Build history of the part. All positions in model axes, mm. Give positions to 0.01 mm unless a question says otherwise; leave off trailing zeros. Loops run counter-clockwise (first coordinate to the right, second up) from the corner with the lowest first, then second, coordinate; pieces in that order, holes last. Notation, with made-up numbers: (26, 68) - (67, 68) arc R24 ccw to (67, 99) - close; hole circle Ø9 at (17.25, 85.25). An arc over 180 degrees is marked (long way). Return JSON: item names as keys, results as strings. Group by question number.
1) Slice it at C-C (y = -4). List the corners of the cut face in (x, z), and give its area (3 significant figures).
2) Slice it at D-D (x = 1.3). Count the separate pieces of the cut face and the enclosed holes in it, and give its area (3 significant figures).
3) Drop flat-ended pins along their axis: pin 1 (20.5 mm diameter, centred on y = -34, z = 0, fed in from -X); pin 2 (1.5 mm diameter, centred on x = 1, y = 31, fed in from -Z); pin 3 (1 mm diameter, centred on x = 0.5, y = 7.5, fed in from -Z). Give the stop position or say it passes through.
4) Drill centre lines: probe 1 along Z at (x, y) = (0.8, -14); probe 2 along Z at (x, y) = (1.15, 44.5); probe 3 along Y at (x, z) = (2.3, 0). Where is each one in solid material? Low to high. Write a range as from..to.
5) Slice it at A-A (y = 42). List the corners of the cut face in (x, z).
6) Slice it at B-B (y = -38). List the corners of the cut face in (x, z), and give its area (3 significant figures).
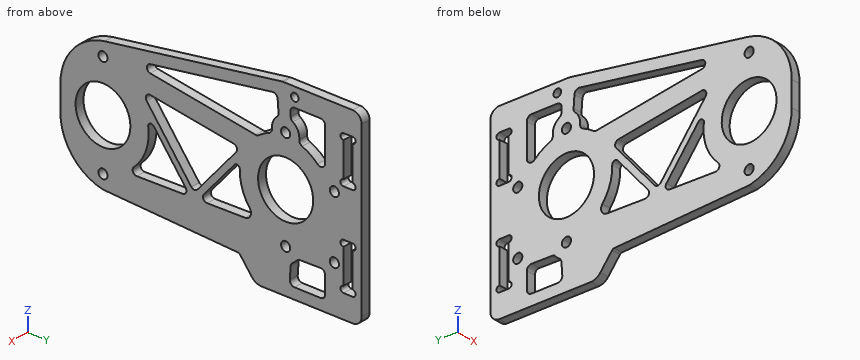
```python
from build123d import *

# Parameters (mm, degrees)
SKETCH_1_W          = 60
SKETCH_1_H          = 96
SKETCH_1_R          = 1.5
SKETCH_1_R_2        = 9
SKETCH_1_R_3        = 9.05
SKETCH_1_H_2        = 3
EXTRUDE_1_DEPTH     = 3
CUT_EXTRUDE_START   = -3
CUT_EXTRUDE_1_DEPTH = 3
SKETCH_3_R          = 1.25
SKETCH_3_R_2        = 1.5
SKETCH_3_W          = 15
SKETCH_3_H          = 3
CUT_EXTRUDE_2_DEPTH = 60.245252974
SKETCH_4_R          = 1
CUT_EXTRUDE_3_DEPTH = 60.245252974
CUT_EXTRUDE_4_DEPTH = 10
CUT_EXTRUDE_5_DEPTH = 60.245252974
EXTRUDE_2_DEPTH     = 3
FILLET_1_R          = 1.3
FILLET_9_R          = 2
FILLET_3_R          = 3
FILLET_4_R          = 1.5
FILLET_5_R          = 4
CUT_EXTRUDE_6_DEPTH = 60.251242528
FILLET_6_R          = 1
FILLET_10_R         = 5


# Read off the part's stored shape, not the designer's step: 切除-拉伸1
with BuildPart() as part:
    # 草图1 → 凸台-拉伸1 (new body)
    # profile 1 of 2: a face of its own
    with BuildSketch(Plane(origin=(0, 0, 0), x_dir=(0, 0, -1), z_dir=(1, 0, 0))):
        Rectangle(SKETCH_1_W, SKETCH_1_H)
        with Locations((16.5, -34)):
            Circle(SKETCH_1_R, mode=Mode.SUBTRACT)
        with Locations((-16.5, -34)):
            Circle(SKETCH_1_R, mode=Mode.SUBTRACT)
        with Locations((16, 26)):
            Circle(SKETCH_1_R, mode=Mode.SUBTRACT)
        with Locations((-16, 26)):
            Circle(SKETCH_1_R, mode=Mode.SUBTRACT)
        with Locations((0, -34)):
            Circle(SKETCH_1_R_2, mode=Mode.SUBTRACT)
        with Locations((0, 26)):
            Circle(SKETCH_1_R_3, mode=Mode.SUBTRACT)
    # profile 2 of 2: a face of its own
    with BuildSketch(Plane(origin=(0, 0, 0), x_dir=(0, 0, -1), z_dir=(1, 0, 0))):
        with Locations((0, 49.5)):
            Rectangle(SKETCH_1_W, SKETCH_1_H_2)
    extrude(amount=EXTRUDE_1_DEPTH)

    # 切除-拉伸1 outline → 切除-拉伸1 (cut)
    with BuildSketch(Plane(origin=(3, 0, 0), x_dir=(0, 0, -1), z_dir=(1, 0, 0)).offset(CUT_EXTRUDE_START)):
        with BuildLine():
            Line((30, -48), (30, 25))
            Line((30, 25), (21, -33.41847233))
            ThreePointArc((21, -33.41847233), (15.198447986, -43.855245061), (4, -48))
            Line((4, -48), (30, -48))
        make_face()
        with BuildLine():
            Line((-30, -48), (-4, -48))
            ThreePointArc((-4, -48), (-15.198447986, -43.855245061), (-21, -33.41847233))
            Line((-21, -33.41847233), (-30, 25))
            Line((-30, 25), (-30, -48))
        make_face()
    extrude(amount=CUT_EXTRUDE_1_DEPTH, mode=Mode.SUBTRACT)

    # 草图3 → 切除-拉伸2 (cut, through all)
    with BuildSketch(Plane(origin=(3, 0, 0), x_dir=(0, 0, -1), z_dir=(1, 0, 0))):
        with Locations((-27, 29)):
            Circle(SKETCH_3_R)
        with Locations((15, 42)):
            Circle(SKETCH_3_R_2)
        with Locations((-5, 42)):
            Circle(SKETCH_3_R_2)
        with Locations((-15, 46.5)):
            Rectangle(SKETCH_3_W, SKETCH_3_H)
        with Locations((15, 46.5)):
            Rectangle(SKETCH_3_W, SKETCH_3_H)
    extrude(amount=-CUT_EXTRUDE_2_DEPTH, mode=Mode.SUBTRACT)

    # 草图4 → 切除-拉伸3 (cut, through all)
    with BuildSketch(Plane(origin=(3, 0, 0), x_dir=(0, 0, -1), z_dir=(1, 0, 0))):
        with Locations((-21.5, 48)):
            Circle(SKETCH_4_R)
        with Locations((-21.5, 45)):
            Circle(SKETCH_4_R)
        with Locations((-8.5, 48)):
            Circle(SKETCH_4_R)
        with Locations((-8.5, 45)):
            Circle(SKETCH_4_R)
        with Locations((8.5, 45)):
            Circle(SKETCH_4_R)
        with Locations((8.5, 48)):
            Circle(SKETCH_4_R)
        with Locations((21.5, 45)):
            Circle(SKETCH_4_R)
        with Locations((21.5, 48)):
            Circle(SKETCH_4_R)
    extrude(amount=-CUT_EXTRUDE_3_DEPTH, mode=Mode.SUBTRACT)

    # 草图6 → 切除-拉伸4 (cut)
    with BuildSketch(Plane(origin=(3, 0, 0), x_dir=(0, 0, -1), z_dir=(1, 0, 0))):
        with BuildLine():
            Line((-18.4613646, -26.910285625), (-11.857625415, 16.731816817))
            ThreePointArc((-11.857625415, 16.731816817), (-13.391258067, 19.13146978), (-14.445390625, 21.777063854))
            ThreePointArc((-14.445390625, 21.777063854), (-17.513828963, 21.762273974), (-19.878390466, 23.71787656))
            Line((-19.878390466, 23.71787656), (-26.191708785, 23.266925251))
            Line((-26.191708785, 23.266925251), (-18.4613646, -26.910285625))
        make_face()
        Polygon((11.318506757, -4.002376427), (-6.62076356, 11.237090825), (-11.596047133, -21.643044091), align=None)
        with BuildLine():
            Line((13.365007146, -27.189964466), (12.932647682, -5.283751611))
            Line((12.932647682, -5.283751611), (-7.478738852, -20.99736699))
            ThreePointArc((-7.478738852, -20.99736699), (4.271897059, -19.621165015), (13.365007146, -27.189964466))
        make_face()
        with BuildLine():
            Line((12.881773753, -2.706139182), (12.481185497, 17.590332433))
            ThreePointArc((12.481185497, 17.590332433), (5.342673899, 11.930233278), (-3.753500841, 11.425579551))
            Line((-3.753500841, 11.425579551), (12.881773753, -2.706139182))
        make_face()
        with BuildLine():
            Line((26.5, 39), (18.059794784, 39))
            Line((18.059794784, 39), (18.239335866, 29.903251834))
            ThreePointArc((18.239335866, 29.903251834), (19.384344521, 28.965840886), (20.163378666, 27.707711359))
            Line((20.163378666, 27.707711359), (26.5, 27.25509555))
            Line((26.5, 27.25509555), (26.5, 39))
        make_face()
        with BuildLine():
            Line((-8.584722927, 38.361433261), (-8.488097697, 39))
            Line((-8.488097697, 39), (-24, 39))
            Line((-24, 39), (-24, 27.433666978))
            Line((-24, 27.433666978), (-20.163378666, 27.707711359))
            ThreePointArc((-20.163378666, 27.707711359), (-17.811907347, 30.119100844), (-14.445390625, 30.222936146))
            ThreePointArc((-14.445390625, 30.222936146), (-12.212915965, 34.794724761), (-8.584722927, 38.361433261))
        make_face()
        with BuildLine():
            ThreePointArc((-8.584722927, 38.361433261), (-8.090184405, 38.690603464), (-7.583040287, 39))
            Line((-7.583040287, 39), (-8.488097697, 39))
            Line((-8.488097697, 39), (-8.584722927, 38.361433261))
        make_face()
    extrude(amount=-CUT_EXTRUDE_4_DEPTH, mode=Mode.SUBTRACT)

    # 草图7 → 切除-拉伸5 (cut, through all)
    with BuildSketch(Plane(origin=(3, 0, 0), x_dir=(0, 0, -1), z_dir=(1, 0, 0))):
        Polygon((28.43912679, 14.868463508), (23.170360519, 10.752052151), (24.727709786, -9.222126667), align=None)
    extrude(amount=-CUT_EXTRUDE_5_DEPTH, mode=Mode.SUBTRACT)

    # 草图8 → 凸台-拉伸2 (add)
    with BuildSketch(Plane(origin=(3, 0, 0), x_dir=(0, 0, -1), z_dir=(1, 0, 0))):
        Polygon((28.43912679, 14.868463508), (30.015148297, 16.099786459), (30, 25), align=None)
    extrude(amount=-EXTRUDE_2_DEPTH)

    # 圆角1
    fillet_1_edges = [part.edges().sort_by_distance(p)[0] for p in [
        (1.5, -2.706139182, -12.881773753),
        (1.5, -4.002376427, -11.318506757),
        (1.5, -21.643044091, 11.596047133),
        (1.5, 11.237090825, 6.62076356),
        (1.5, -27.189964466, -13.365007146),
        (1.5, -5.283751611, -12.932647682),
        (1.5, -26.910285625, 18.4613646),
    ]]
    fillet(fillet_1_edges, radius=FILLET_1_R)

    # 圆角9
    fillet_9_edges = [part.edges().sort_by_distance(p)[0] for p in [
        (1.5, 17.590332433, -12.481185497),
    ]]
    fillet(fillet_9_edges, radius=FILLET_9_R)

    # 圆角3
    fillet_3_edges = [part.edges().sort_by_distance(p)[0] for p in [
        (1.5, 51, 30),
        (1.5, 51, -30),
        (1.5, 25, 30),
    ]]
    fillet(fillet_3_edges, radius=FILLET_3_R)

    # 圆角4
    fillet_4_edges = [part.edges().sort_by_distance(p)[0] for p in [
        (1.5, 27.707711359, -20.163378666),
        (1.5, 29.903251834, -18.239335866),
        (1.5, 39, -18.059794784),
        (1.5, 39, -26.5),
        (1.5, 27.25509555, -26.5),
        (1.5, 30.222936146, 14.445390625),
        (1.5, 27.707711359, 20.163378666),
        (1.5, 27.433666978, 24),
        (1.5, 39, 24),
        (1.5, 39, 7.583040287),
        (1.5, 23.71787656, 19.878390466),
        (1.5, 21.777063854, 14.445390625),
        (1.5, 16.731816817, 11.857625415),
        (1.5, 23.266925251, 26.191708785),
    ]]
    fillet(fillet_4_edges, radius=FILLET_4_R)

    # 圆角5
    fillet_5_edges = [part.edges().sort_by_distance(p)[0] for p in [
        (1.5, 16.099786459, -30.015148297),
    ]]
    fillet(fillet_5_edges, radius=FILLET_5_R)

    # 草图9 → 切除-拉伸6 (cut, through all)
    with BuildSketch(Plane(origin=(3, 0, 0), x_dir=(0, 0, -1), z_dir=(1, 0, 0))):
        Polygon((23.170360519, 10.752052151), (20.910409348, -34), (24.727709786, -9.222126667), align=None)
    extrude(amount=-CUT_EXTRUDE_6_DEPTH, mode=Mode.SUBTRACT)

    # 圆角6
    fillet_6_edges = [part.edges().sort_by_distance(p)[0] for p in [
        (1.5, 11.425579551, 3.753500841),
        (1.5, -20.99736699, 7.478738852),
        (1.5, 10.752052151, -23.170360519),
    ]]
    fillet(fillet_6_edges, radius=FILLET_6_R)

    # 圆角10
    fillet_10_edges = [part.edges().sort_by_distance(p)[0] for p in [
        (1.5, -33.925032861, -20.914195142),
    ]]
    fillet(fillet_10_edges, radius=FILLET_10_R)


solid = part.part
```
Results:
{
 "1": {"outline": "(0, -22.43) - (3, -22.43) - (3, -10.55) - (0, -10.55) - close; (0, 8.93) - (3, 8.93) - (3, 14.99) - (0, 14.99) - close; (0, 21.99) - (3, 21.99) - (3, 25.53) - (0, 25.53) - close", "area": "64.5 mm2"},
 "2": {"separate pieces": "1", "enclosed holes": "17", "area": "3,100 mm2"},
 "3": {"pin 1": "x = 0", "pin 2": "z = -30", "pin 3": "z = -23.03"},
 "4": {"probe 1": "-21.92..-13.1, -1.61..1.67, 10.44..16.51, 20.45..23.99", "probe 2": "-30..-22.37, -20.63..-9.37, -7.63..7.63, 9.37..20.63, 22.37..30", "probe 3": "-48..-43, -25..-19, -15.24..-12.72, 5.61..8.24, 10.95..16.95, 35.05..51"},
 "5": {"outline": "(0, -30) - (3, -30) - (3, -16.5) - (0, -16.5) - close; (0, -13.5) - (3, -13.5) - (3, 3.5) - (0, 3.5) - close; (0, 6.5) - (3, 6.5) - (3, 30) - (0, 30) - close"},
 "6": {"outline": "(0, -19.62) - (3, -19.62) - (3, -8.06) - (0, -8.06) - close; (0, 8.06) - (3, 8.06) - (3, 19.62) - (0, 19.62) - close", "area": "69.4 mm2"}
}
